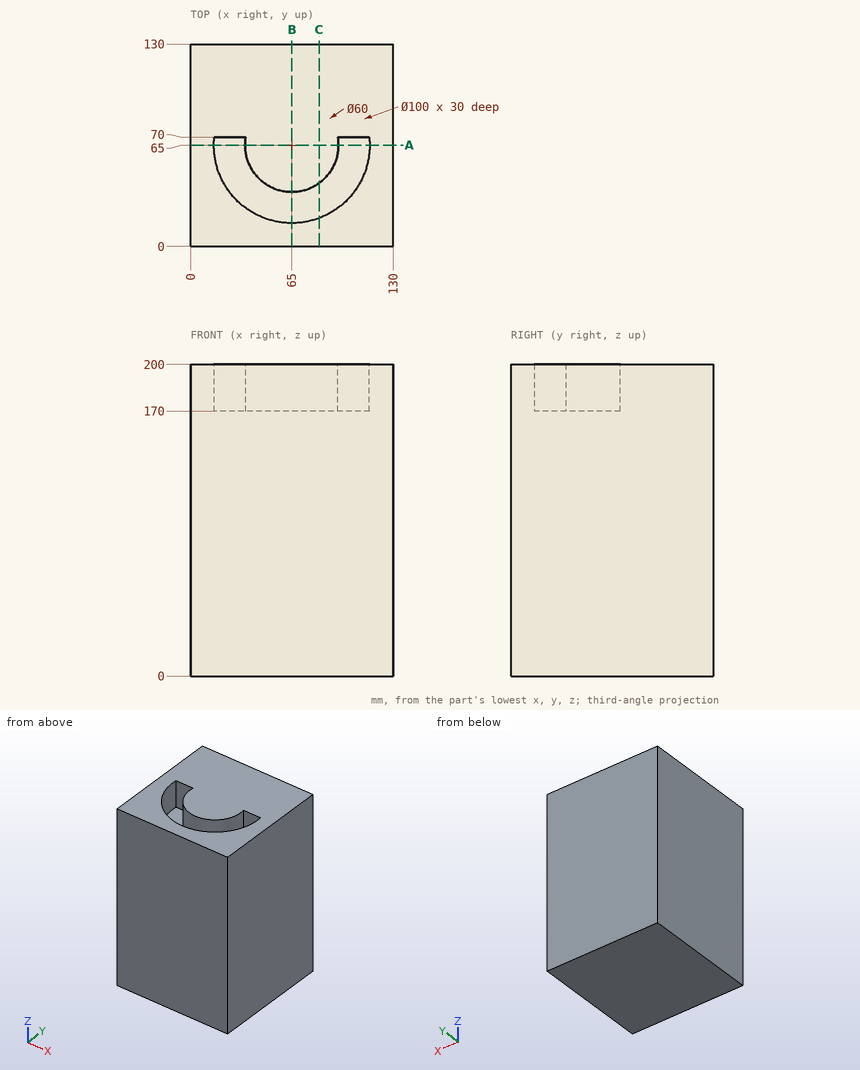
Study the drawing (mm; zero at the part's minimum x, y, z) and answer. Give positions to 0.01 mm unless a question says otherwise; leave off trailing zeros. Order: outer loops, then holes, each group sorted by start corner. A loop starts at its lowest first (then second) coordinate and runs counter-clockwise, first axis right, second up. Notation, with made-up numbers: (-30, 76.5) - (2, 76.5) arc R21 ccw to (2, 89.5) - close; hole circle Ø3 at (19.5, -6.75). An arc over 180 degrees is marked (long way). Answer in a Markdown table with one row per item. Add a question column.
Q1. Given P1, Ø10, axis at y = 86.5, z = 73.5, coming from the -X side; P2, Ø3, axis at x = 37, y = 28.5, coming from the +Z side, each flat-ended and moving along its own axis, determine where each tip first touches the part or whether it passes through.
Q2. The part is cut by section C-C (x = 82.5). Determine the outline of the cut face in (y, z), then the cut area to 3 significant figures.
Q3. Find the intervals of material crossed by line 1 along X through (y, z) = (65, 181); line 2 along X through (y, z) = (30.5, 173), in increasing order. Write a range as [from, to].
Q4. The part is cut by section A-A (y = 65). Determine the outline of the cut face in (x, z), then the cut area to 3 significant figures.
Q5. The part is cut by section B-B (x = 65). Determine the outline of the cut face in (y, z), then the cut area to 3 significant figures.
Determined:
| question | item | result |
|---|---|---|
| 1 | P1 | stops at x = 0 |
| 1 | P2 | stops at z = 170 |
| 2 | outline | (0, 0) - (130, 0) - (130, 200) - (40.63, 200) - (40.63, 170) - (18.16, 170) - (18.16, 200) - (0, 200) - close |
| 2 | area | 25,300 mm² |
| 3 | line 1 | x = [0, 15], [35, 95], [115, 130] |
| 3 | line 2 | x = [0, 28.81], [101.19, 130] |
| 4 | outline | (0, 0) - (130, 0) - (130, 200) - (115, 200) - (115, 170) - (95, 170) - (95, 200) - (35, 200) - (35, 170) - (15, 170) - (15, 200) - (0, 200) - close |
| 4 | area | 24,800 mm² |
| 5 | outline | (0, 0) - (130, 0) - (130, 200) - (35, 200) - (35, 170) - (15, 170) - (15, 200) - (0, 200) - close |
| 5 | area | 25,400 mm² |
